```python
from build123d import *

# Parameters (mm, degrees)
SKETCH1_R            = 1.53035
BOSS_EXTRUDE1_DEPTH  = 50.8
BOSS_EXTRUDE2_DEPTH  = 0.508
MIRROR2_COPY_1_DEPTH = 0.508


with BuildPart() as part:
    # Sketch1 → Boss-Extrude1 (new body)
    with BuildSketch(Plane.XY):
        Circle(SKETCH1_R)
    extrude(amount=BOSS_EXTRUDE1_DEPTH)

    # Sketch2 → Boss-Extrude2 (add, symmetric)
    with BuildSketch(Plane(origin=(0, 0, 0), x_dir=(0, 0, -1), z_dir=(1, 0, 0))):
        with BuildLine():
            ThreePointArc((-46.99, 1.14935), (-48.26, 2.41935), (-49.53, 1.14935))
            Line((-49.53, 1.14935), (-49.276, 1.14935))
            ThreePointArc((-49.276, 1.14935), (-48.26, 2.16535), (-47.244, 1.14935))
            Line((-47.244, 1.14935), (-46.99, 1.14935))
        make_face()
    boss_extrude2 = extrude(amount=BOSS_EXTRUDE2_DEPTH, both=True)

    # Mirror1: Boss-Extrude2 across plane
    add(boss_extrude2.mirror(Plane.ZX))

    # Mirror2: Boss-Extrude2 across plane
    add(boss_extrude2.mirror(Plane(origin=(0, 0, 25.4), x_dir=(1, 0, 0), z_dir=(0, 0, -1))))

    # Mirror2 copy 1 sketch → Mirror2 copy 1 (add, symmetric)
    with BuildSketch(Plane(origin=(0, 0, 50.8), x_dir=(0, 0, 1), z_dir=(1, 0, 0))):
        with BuildLine():
            ThreePointArc((-46.99, 1.14935), (-48.26, 2.41935), (-49.53, 1.14935))
            Line((-49.53, 1.14935), (-49.276, 1.14935))
            ThreePointArc((-49.276, 1.14935), (-48.26, 2.16535), (-47.244, 1.14935))
            Line((-47.244, 1.14935), (-46.99, 1.14935))
        make_face()
    extrude(amount=MIRROR2_COPY_1_DEPTH, both=True)


solid = part.part
```
Could you check a few things on this model? Use its own coordinates, in mm. A direction names the side the tool comes from. Give positions to 0.01 mm unless a question says otherwise; leave off trailing zeros. Loops run counter-clockwise (first coordinate to the right, second up) from the corner with the lowest first, then second, coordinate; pieces in that order, holes last. Notation, with made-up numbers: (-28.5, 21) - (21.5, 21) arc R23 cw to (21.5, 57) - close; hole circle Ø8 at (-7, 83). An arc over 180 degrees is marked (long way). Answer in a Markdown table with one row per item. Add a question column.
Q1. If we section it at A-A (x = 0): List the corners of the cut face in (y, z) for me.
Q2. Which directions (+Z, -Z, +X, -X, +Y, -Y) give clear straight access to the entire face, cutting with the end or side of a thin tool? Please do faces 4 (the face through (0, 0, 50.8)), 5 (the face through (-0.3, -1.5, 25)).
Q3. If we section it at B-B (z = 15.5): List the corners of the cut face in (x, y) for me.
Q4. We'd pull the mould along Y, two halves only. Please class faces 1 (the face through (0.01, 2.42, 48.24)), 2 (the face through (0, 0, 0)), 3 (the face through (0.007, 2.165, 2.522)): +Y half, -Y half, draft (parallel to the pull), parting line (faces both ways), or undercut.
Q5. For pin 1 (1.1 mm diameter, centred on y = 1.5, z = 2, fed in from +X); pin 2 (0.8 mm diameter, centred on y = 1.5, z = 2.5, fed in from -X); pin 3 (0.8 mm diameter, centred on y = 2, z = 48.5, fed in from -X), each with a flat end and sliding along its axis, tell me the tip position at first contact or that it passes through.
Q6. If we section it at C-C (y = -0.55): List the corners of the cut face in (x, z) for me.
Q7. Please list where these lines run through material, in increasing order: L1, parallel to Z at x = 0.05, y = 1.6; L2, parallel to Y at x = -0.1, z = 19.5; L3, parallel to Z at x = 0, y = 1.9. Write a range as from..to.
The answers:
| question | item | result |
|---|---|---|
| 1 | outline | (-1.53, 0) - (1.53, 0) - (1.53, 1.33) arc R1.27 ccw to (1.53, 3.75) - (1.53, 47.05) arc R1.27 ccw to (1.53, 49.47) - (1.53, 50.8) - (-1.53, 50.8) - (-1.53, 49.47) arc R1.27 ccw to (-1.53, 47.05) - (-1.53, 3.75) arc R1.27 ccw to (-1.53, 1.33) - close; hole (-1.53, 1.6) - (-1.53, 3.48) arc R1.02 ccw to start; hole (-1.53, 47.32) - (-1.53, 49.2) arc R1.02 ccw to start; hole (1.53, 1.6) arc R1.02 ccw to (1.53, 3.48) - close; hole (1.53, 47.32) arc R1.02 ccw to (1.53, 49.2) - close |
| 2 | face 4 | +Z, +X, -X, +Y, -Y |
| 2 | face 5 | none |
| 3 | outline | circle Ø3.06 at (0, 0) |
| 4 | face 1 | +Y half |
| 4 | face 2 | draft |
| 4 | face 3 | undercut |
| 5 | pin 1 | stops at x = 1.2 |
| 5 | pin 2 | stops at x = -1.06 |
| 5 | pin 3 | stops at x = -0.51 |
| 6 | outline | (-1.43, 0) - (1.43, 0) - (1.43, 50.8) - (-1.43, 50.8) - close |
| 7 | L1 | z = 1.35..1.63, 3.45..3.73, 47.07..47.35, 49.17..49.45 |
| 7 | L2 | y = -1.53..1.53 |
| 7 | L3 | z = 1.52..1.86, 3.22..3.56, 47.24..47.58, 48.94..49.28 |
